Here's the drawing with two shaded views (mm, measured from the low corner). I have some questions. Coordinates: 2 decimals unless noted, no trailing zeros. Order: outer loops, then holes, each group sorted by start corner. A loop starts at its lowest first (then second) coordinate and runs counter-clockwise, first axis right, second up. Notation, with made-up numbers: (43.5, -14) -> (84.5, -14) arc R14 cw to (84.5, -8) -> close; hole circle Ø8 at (69, 30.25). An arc over 180 degrees is marked (long way). Write item = value, one per line.
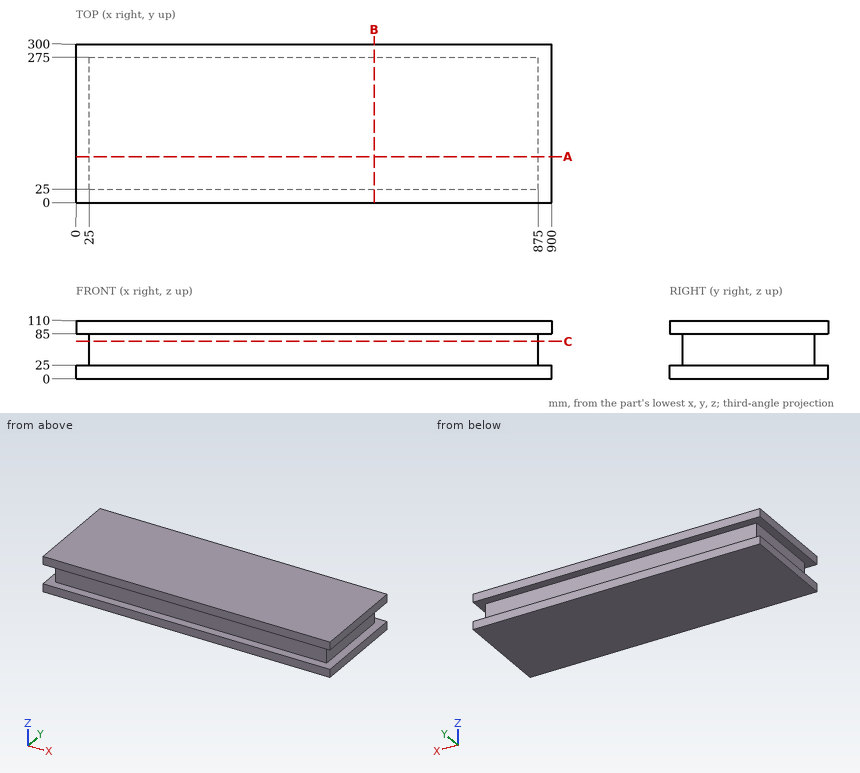
Item 1: I want a section at B-B, the plane x = 564.5. Please give me the cut outline in (y, z), plus the area to 3 significant figures.
A:
outline = (0, 0) -> (300, 0) -> (300, 25) -> (275, 25) -> (275, 85) -> (300, 85) -> (300, 110) -> (0, 110) -> (0, 85) -> (25, 85) -> (25, 25) -> (0, 25) -> close
area = 30,000 mm2
Item 2: If I drill on probe 1 along Z at (x, y) = (517, 19); probe 2 along Y at (x, z) = (225.5, 28); probe 3 along X at (y, z) = (164, 74), over which ranges is the centre line in solid material (lowest first)?
A:
probe_1 = 0 to 25, 85 to 110
probe_2 = 25 to 275
probe_3 = 25 to 875
Item 3: I want a section at C-C, the plane z = 70.5. Please give me the cut outline in (x, y), plus the area to 4 significant figures.
A:
outline = (25, 25) -> (875, 25) -> (875, 275) -> (25, 275) -> close
area = 212,500 mm2
Item 4: I want a section at A-A, the plane y = 87. Please give me the cut outline in (x, z).
A:
outline = (0, 0) -> (900, 0) -> (900, 25) -> (875, 25) -> (875, 85) -> (900, 85) -> (900, 110) -> (0, 110) -> (0, 85) -> (25, 85) -> (25, 25) -> (0, 25) -> close
Item 5: I'm going to push flat-ended pins straight in: P1, Ø4, axis at x = 762, z = 91.5, coming from the -Y side; P2, Ø1.5, axis at y = 54, z = 82.5, coming from the +X side; P3, Ø1.5, axis at x = 522, z = 56.5, coming from the -Y side; P4, Ø1.5, axis at y = 84.5, z = 60, coming from the -X side. Where does each tip first touch, or does it pass through?
A:
P1 = 0
P2 = 875
P3 = 25
P4 = 25
